Geometry check sheet. Reference: the model listing, model coordinates, mm. A direction names the side the tool comes from. Give positions to 0.01 mm unless a question says otherwise; leave off trailing zeros. Order: outer loops, then holes, each group sorted by start corner. A loop starts at its lowest first (then second) coordinate and runs counter-clockwise, first axis right, second up. Notation, with made-up numbers: M 78.25,76 L 99.25,76 A17 ccw 99.25,109 Z; hole C 16,-20 d5. An arc over 180 degrees is marked long. Answer as CSV lines item,"result".
from build123d import *

# Parameters (mm, degrees)
SKETCH1_R           = 1.3890625
BOSS_EXTRUDE1_DEPTH = 6.35


with BuildPart() as part:
    # Sketch1 → Boss-Extrude1 (new body)
    with BuildSketch(Plane.XY):
        with BuildLine():
            Line((12.7, 0), (-12.7, 0))
            Line((-12.7, 0), (-12.7, -16.51))
            ThreePointArc((-12.7, -16.51), (-13.443948776, -18.306051224), (-15.24, -19.05))
            Line((-15.24, -19.05), (-25.4, -19.05))
            ThreePointArc((-25.4, -19.05), (-29.21, -15.24), (-25.4, -11.43))
            ThreePointArc((-25.4, -11.43), (-20.909871939, -9.570128061), (-19.05, -5.08))
            Line((-19.05, -5.08), (-19.05, 1.27))
            add(Edge.make_bspline(
                [(-19.05, 1.27), (-19.05, 15.828620542), (-38.807847876, 23.500433408)],
                knots=[0, 0, 0, 1.015776501, 1.015776501, 1.015776501], degree=2, weights=[1, 0.873773469, 1]))
            ThreePointArc((-38.807847876, 23.500433408), (-41.155413928, 30.410828457), (-33.941740139, 31.518771801))
            ThreePointArc((-33.941740139, 31.518771801), (0, 18.732499831), (33.941740139, 31.518771801))
            ThreePointArc((33.941740139, 31.518771801), (41.155413928, 30.410828457), (38.807847876, 23.500433408))
            add(Edge.make_bspline(
                [(38.807847876, 23.500433408), (19.05, 15.828620542), (19.05, 1.27)],
                knots=[2.125816153, 2.125816153, 2.125816153, 3.141592654, 3.141592654, 3.141592654], degree=2, weights=[1, 0.873773469, 1]))
            Line((19.05, 1.27), (19.05, -5.08))
            ThreePointArc((19.05, -5.08), (20.909871939, -9.570128061), (25.4, -11.43))
            ThreePointArc((25.4, -11.43), (29.21, -15.24), (25.4, -19.05))
            Line((25.4, -19.05), (15.24, -19.05))
            ThreePointArc((15.24, -19.05), (13.443948776, -18.306051224), (12.7, -16.51))
            Line((12.7, -16.51), (12.7, 0))
        make_face()
        with Locations((-37.084, 27.94)):
            Circle(SKETCH1_R, mode=Mode.SUBTRACT)
        with Locations((-25.4, -15.24)):
            Circle(SKETCH1_R, mode=Mode.SUBTRACT)
        with Locations(Location((25.4, -15.24, 0), (0, 0, 180))):
            Circle(SKETCH1_R, mode=Mode.SUBTRACT)
        with Locations(Location((37.084, 27.94, 0), (0, 0, 180))):
            Circle(SKETCH1_R, mode=Mode.SUBTRACT)
    extrude(amount=BOSS_EXTRUDE1_DEPTH)


solid = part.part
(1) Tool access check on faces 4 (the face through (13.464, -18.326, 3.131)), 5 (the face through (1, 7, 0)), 6 (the face through (-19.05, -2, 3)), 7 (the face through (19.05, -2, 3)). Record the directions out of +Z, -Z, +X, -X, +Y, -Y that give a thin tool (end or side, any length) a straight path to the whole face; none if there is none.
The answers:
face 4,"+Z, -Z, -Y"
face 5,"-Z, +X, -X, +Y, -Y"
face 6,"+Z, -Z, -X"
face 7,"+Z, -Z, +X"
(2) Section check A-A on y = -15.24. Enter the section's corners in (x, z).
The answers:
outline,"M -29.21,0 L -26.79,0 L -26.79,6.35 L -29.21,6.35 Z; M -24.01,0 L -12.7,0 L -12.7,6.35 L -24.01,6.35 Z; M 12.7,0 L 24.01,0 L 24.01,6.35 L 12.7,6.35 Z; M 26.79,0 L 29.21,0 L 29.21,6.35 L 26.79,6.35 Z"
(3) Material ranges on line 1 (Y direction, x = -25.4, z = 5); line 2 (X direction, y = -4, z = 5.25); line 3 (X direction, y = -5.5, z = 2.5), recorded low to high.
The answers:
line 1,"y = -19.05 to -16.63, -13.85 to -11.43, 15.13 to 25.44"
line 2,"x = -19.05 to -12.7, 12.7 to 19.05"
line 3,"x = -19.06 to -12.7, 12.7 to 19.06"
(4) Gauge pin test, flat ends, axial feed: P1, Ø2, axis at x = 25.4, y = -15.24, coming from the -Z side; P2, Ø3, axis at x = 1, z = 3.5, coming from the -Y side; P3, Ø2, axis at x = 25, z = 1, coming from the +Y side; P4, Ø1.9, axis at y = -9.5, z = 4, coming from the +X side. Record the tip position at first contact, or that the pin passes through.
The answers:
P1,"passes through"
P2,"stops at y = 0"
P3,"stops at y = 25.79"
P4,"stops at x = 22.01"
(5) Section check C-C on z = 1. State how many separate pieces and enclosed holes the cut face has, then the cut area to 3 significant figures.
The answers:
separate pieces,"1"
enclosed holes,"4"
area,"1,600 mm2"
(6) Section check B-B on y = -2.5. Enter the section's corners in (x, z).
The answers:
outline,"M -19.05,0 L -12.7,0 L -12.7,6.35 L -19.05,6.35 Z; M 12.7,0 L 19.05,0 L 19.05,6.35 L 12.7,6.35 Z"
(7) Section check D-D on x = 18. Enter the section's corners in (y, z).
The answers:
outline,"M -19.05,0 L 21.98,0 L 21.98,6.35 L -19.05,6.35 Z"
(8) Draft check along X on faces 1 (the face through (1, 7, 6.35)), 2 (the face through (29.21, -15.16, 3.13)), 3 (the face through (37.385, 29.296, 3.131)). Enter one of: +X half, -X half, draft (parallel to the pull), parting line (faces both ways), or undercut.
The answers:
face 1,"draft"
face 2,"+X half"
face 3,"undercut"
